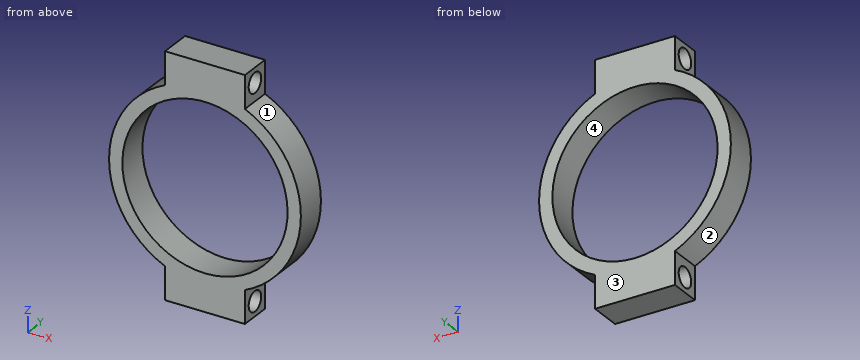
```python
from build123d import *

# Parameters (mm, degrees)
SKETCH1_R           = 39.37
BOSS_EXTRUDE1_DEPTH = 15.24
SKETCH2_R           = 4.7625
CUT_EXTRUDE1_DEPTH  = 88.712786981


with BuildPart() as part:
    # Sketch1 → Boss-Extrude1 (new body)
    with BuildSketch(Plane(origin=(0, 0, 0), x_dir=(1, 0, 0), z_dir=(0, 1, 0))):
        with BuildLine():
            Line((-19.05, 57.15), (19.05, 57.15))
            Line((19.05, 57.15), (19.05, 41.562193157))
            ThreePointArc((19.05, 41.562193157), (45.72, 0), (19.05, -41.562193157))
            Line((19.05, -41.562193157), (19.05, -57.15))
            Line((19.05, -57.15), (-19.05, -57.15))
            Line((-19.05, -57.15), (-19.05, -41.562193157))
            ThreePointArc((-19.05, -41.562193157), (-45.72, 0), (-19.05, 41.562193157))
            Line((-19.05, 41.562193157), (-19.05, 57.15))
        make_face()
        with Locations(Location((0, 0, 0), (0, 0, 90))):
            Circle(SKETCH1_R, mode=Mode.SUBTRACT)
    extrude(amount=BOSS_EXTRUDE1_DEPTH)

    # Sketch2 → Cut-Extrude1 (cut, through all)
    with BuildSketch(Plane.ZY.offset(19.05)):
        with BuildLine():
            ThreePointArc((45.4025, 7.62), (50.165, 2.8575), (54.9275, 7.62))
            Line((54.9275, 7.62), (45.4025, 7.62))
        make_face()
        with BuildLine():
            Line((45.4025, 7.62), (54.9275, 7.62))
            ThreePointArc((54.9275, 7.62), (50.165, 12.3825), (45.4025, 7.62))
        make_face()
        with Locations((-50.165, 7.62)):
            Circle(SKETCH2_R)
    extrude(amount=-CUT_EXTRUDE1_DEPTH, mode=Mode.SUBTRACT)


solid = part.part
```
Can you work these out from the model? Positions are in its coordinate system, mm. Face numbers are marked on the shaded views. Coordinates: 2 decimals unless noted, no trailing zeros. Loops run counter-clockwise (first coordinate to the right, second up) from the corner with the lowest first, then second, coordinate; pieces in that order, holes last.
Item 1: Suppose I cut it at A-A (y = 7.62). Please give me the cut outline in (x, z).
Answers below:
outline: (-19.05, -57.15) - (19.05, -57.15) - (19.05, -54.93) - (-19.05, -54.93) - close; (-19.05, -45.4) - (19.05, -45.4) - (19.05, -41.56) arc R45.72 ccw to (19.05, 41.56) - (19.05, 45.4) - (-19.05, 45.4) - (-19.05, 41.56) arc R45.72 ccw to (-19.05, -41.56) - close; (-19.05, 54.93) - (19.05, 54.93) - (19.05, 57.15) - (-19.05, 57.15) - close; hole circle Ø78.74 at (0, 0)
Item 2: Suppose I cut it at D-D (x = -37). Please give me the cut outline in (y, z).
Answers below:
outline: (0, -26.86) - (15.24, -26.86) - (15.24, -13.45) - (0, -13.45) - close; (0, 13.45) - (15.24, 13.45) - (15.24, 26.86) - (0, 26.86) - close
Item 3: I'm going to push flat-ended pins straight in: pin 1 (4.5 mm diameter, centred on y = 8, z = 50.5, fed in from -X); pin 2 (7.5 mm diameter, centred on y = 8, z = -51.5, fed in from -X); pin 3 (5 mm diameter, centred on y = 6, z = -16, fed in from +X); pin 4 (6 mm diameter, centred on x = -24.5, y = 4, fed in from -Z). Where does each tip first touch, or does it pass through?
Answers below:
pin 1: passes through
pin 2: stops at x = -19.05
pin 3: stops at x = 43.68
pin 4: stops at z = -40.35
Item 4: Please list where these lines run through material, in increasing order: L1, parallel to X at y = 11.5, z = 0; L2, parallel to Z at x = -7.5, y = 8; L3, parallel to Z at x = -24.5, y = 3.25.
Answers below:
L1: x = -45.72 to -39.37, 39.37 to 45.72
L2: z = -57.15 to -54.91, -45.42 to -38.65, 38.65 to 45.42, 54.91 to 57.15
L3: z = -38.6 to -30.82, 30.82 to 38.6
Item 5: Suppose I cut it at C-C (z = 37.5). Please give me the cut outline in (x, y).
Answers below:
outline: (-26.15, 0) - (-11.99, 0) - (-11.99, 15.24) - (-26.15, 15.24) - close; (11.99, 0) - (26.15, 0) - (26.15, 15.24) - (11.99, 15.24) - close
Item 6: If we mould it in two halves opening along X, with no side actions, what happens to the marked faces 1, 2, 3 and 4? For each: released by +X, released by -X, zero draft, split by the parting line, or undercut.
Answers below:
face 1: released by +X
face 2: released by -X
face 3: zero draft
face 4: undercut
Item 7: Suppose I cut it at B-B (x = 0). State how many separate pieces and enclosed holes the cut face has, then the cut area to 3 significant figures.
Answers below:
separate pieces: 2
enclosed holes: 2
area: 399 mm2
